Input: part model. Units: mm. Frame: model coordinates. A direction names the side the tool comes from. Coordinates: 2 decimals unless noted, no trailing zeros. Order: outer loops, then holes, each group sorted by start corner. A loop starts at its lowest first (then second) coordinate and runs counter-clockwise, first axis right, second up.
from build123d import *

# Parameters (mm, degrees)
SKETCH1_W           = 71.12
SKETCH1_H           = 76.2
BOSS_EXTRUDE1_DEPTH = 50.038
SKETCH2_W           = 1.27
SKETCH2_H           = 50.038
BOSS_EXTRUDE2_DEPTH = 12.7
SKETCH3_R           = 1.5875
CUT_EXTRUDE1_DEPTH  = 80.680330346


with BuildPart() as part:
    # Sketch1 → Boss-Extrude1 (new body)
    with BuildSketch(Plane(origin=(0, 0, 0), x_dir=(1, 0, 0), z_dir=(0, 1, 0))):
        Rectangle(SKETCH1_W, SKETCH1_H)
    extrude(amount=BOSS_EXTRUDE1_DEPTH)

    # Sketch2 → Boss-Extrude2 (add)
    with BuildSketch(Plane(origin=(0, 0, -38.1), x_dir=(-1, 0, 0), z_dir=(0, 0, -1))):
        with Locations((34.925, 25.019)):
            Rectangle(SKETCH2_W, SKETCH2_H)
    extrude(amount=BOSS_EXTRUDE2_DEPTH)

    # Sketch3 → Cut-Extrude1 (cut, through all)
    with BuildSketch(Plane.XZ):
        with Locations(Location((0.762, 1.778, 0), (0, 0, 270))):
            Circle(SKETCH3_R)
    extrude(amount=-CUT_EXTRUDE1_DEPTH, mode=Mode.SUBTRACT)


solid = part.part
Item 1: Access query for faces 1 (the face through (0, 25, -38.1)), 2 (the face through (0, 0, -6)). Directions: +Z, -Z, +X, -X, +Y, -Y. A direction counts if a zero-diameter tool reaches every point of the face in a straight line with its end or side. Return the directions, or none.
Response values:
face 1: -Z, +X, +Y, -Y
face 2: +Z, -Z, +X, -X, -Y
Item 2: Ray query, probe 1 along Z at (x, y) = (15, 38.5); probe 2 along X at (y, z) = (22.5, 0.5). Return the intervals inside material, ascending.
Response values:
probe 1: z = -38.1 to 38.1
probe 2: x = -35.56 to -0.18, 1.7 to 35.56
Item 3: Cut plane A-A on y = 22.5. Return loops of the section in (x, z) (1 decimal).
Response values:
outline: (-35.6, -50.8) - (-34.3, -50.8) - (-34.3, -38.1) - (35.6, -38.1) - (35.6, 38.1) - (-35.6, 38.1) - close; hole circle Ø3.2 at (0.8, 1.8)
Item 4: Pin query (flat end, axial travel): pin 1 Ø6.5 at (y, z) = (26.5, -44.5) entering from +X. Return the tip coordinate at first contact, or that it passes through.
Response values:
pin 1: stops at x = -34.29
Item 5: Draft query along Z for faces 3 (the face through (-0.2, 24.67, 3.04)), 4 (the face through (-34.29, 25, -44)), 5 (the face through (0, 25, 38.1)). Return one class per face: pulls with the +Z half, pulls with the -Z half, needs draft (parallel to the pull), parting line crosses it, or undercut.
Response values:
face 3: undercut
face 4: needs draft
face 5: pulls with the +Z half
Item 6: Cut plane B-B on x = 25.5. Return loops of the section in (y, z).
Response values:
outline: (0, -38.1) - (50.04, -38.1) - (50.04, 38.1) - (0, 38.1) - close
